Geometry: final body of the model. Coordinates: model frame, mm. A direction names the side the tool comes from. Give positions to 0.01 mm unless a question says otherwise; leave off trailing zeros. Write each loop counter-clockwise with the first axis right and the second up, starting at its lowest first coordinate (ties: lowest second). Pieces come first, ordered by that corner, then holes. Notation, with made-up numbers: (24, 5) - (39, 5) arc R8 ccw to (39, 17) - close; hole circle Ø11 at (-29.5, 36). An arc over 180 degrees is marked (long way). Return JSON: item names as keys, results as strings.
Autodesk Inventor part; units mm, degrees
ref_plane "Work Plane2" through (0, 0, -30) normal (0, 0, 1) x (1, 0, 0)
ref_plane "Work Plane3" through (45, 0, 0) normal (1, 0, 0) x (0, 1, 0)
ref_plane "XZ Plane" through (0, 0, 0) normal (0, 1, 0) x (-1, 0, 0)
sketch "Sketch1" plane through (0, 0, 0) normal (0, 1, 0) x (-1, 0, 0)
  line L0 (0, 0) -> (-90, 0)
  line L1 (-90, 0) -> (-90, -60)
  line L2 (-90, -60) -> (0, -60)
  line L3 (0, -60) -> (0, 0)
  line L4 (-30, 0) -> (-60, 0)
  line L5 (-60, 0) -> (-60, -60)
  line L6 (-60, -60) -> (-30, -60)
  line L7 (-30, -60) -> (-30, 0)
  line L8 (-20, -60) -> (-70, -60)
  line L9 (-70, -60) -> (-70, 0)
  line L10 (-70, 0) -> (-20, 0)
  line L11 (-20, 0) -> (-20, -60)
  line L12 (-20, -60) -> (-70, -60)
  line L13 (-70, -60) -> (-70, -40)
  line L14 (-70, -40) -> (-20, -40)
  line L15 (-20, -40) -> (-20, -60)
  circle A0 centre (-10, -50) radius 2.75
  circle A1 centre (-10, -10) radius 2.75
  circle A2 centre (-80, -50) radius 2.75
  circle A3 centre (-80, -10) radius 2.75
  point P0 (0, -30)
  point P1 (-60, -40)
  point P2 (-30, -40)
  point P3 (-70, 0)
  point P4 (-20, 0)
  dimension "d0" = 90
  dimension "d1" = 60
  dimension "d2" = 30
  dimension "d3" = 30
  dimension "d4" = 50
  dimension "d5" = 60
  dimension "d6" = 20
  dimension "d7" = 20
  dimension "d8" = 5.5
  dimension "d9" = 5.5
  dimension "d10" = 5.5
  dimension "d11" = 5.5
  dimension "d12" = 10
  dimension "d13" = 10
  dimension "d14" = 10
  dimension "d15" = 10
  dimension "d16" = 10
  dimension "d17" = 10
  dimension "d18" = 10
  dimension "d19" = 10
extrude "Extrusion1" add sketch "Sketch1" along normal blind 10 contours L3 L2 L11 L0 | L9 L2 L1 L0
extrude "Extrusion2" add sketch "Sketch1" along normal blind 20 contours L11 L14 L7 L0 | L7 L14 L5 L0 | L11 L2 L7 L14 | L5 L14 L9 L0 | L5 L2 L9 L14
extrude "Extrusion3" add sketch "Sketch1" along normal blind 50 contours L11 L2 L7 L14 | L7 L2 L5 L14 | L5 L2 L9 L14
extrude "Extrusion4" cut sketch "Sketch1" along normal blind 10 contours L7 L14 L5 L0 | L7 L2 L5 L14
ref_plane "Work Plane2" through (0, 0, -30) normal (0, 0, 1) x (1, 0, 0)
ref_plane "Work Plane3" through (45, 0, 0) normal (1, 0, 0) x (0, 1, 0)
sketch "Sketch7" plane through (0, 0, -30) normal (0, 0, 1) x (1, 0, 0)
  line L0 (20, 10) -> (20, 20)
  line L1 (20, 10) -> (0, 10)
  line L2 (20, 20) -> (0, 10)
  line L3 (0, 10) -> (20, 10)
  line L4 (20, 10) -> (20, 20)
  line L5 (70, 20) -> (60, 20)
  line L6 (70, 20) -> (90, 10)
  line L7 (90, 10) -> (70, 10)
  line L8 (90, 10) -> (70, 10)
  line L9 (70, 10) -> (70, 20)
  point P0 (0, 0)
extrude "Extrusion9" add sketch "Sketch7" along normal mid plane 4
sketch "Sketch8" plane through (45, 0, 0) normal (1, 0, 0) x (0, 1, 0)
  circle A0 centre (40, -50) radius 2.75
  line L0 (20, 0) -> (50, -51.9582)
  line L1 (20, 0) -> (20, -51.9582)
  line L2 (20, -51.9582) -> (50, -51.9582)
  point P0 (0, 0)
  point P1 (38.0692, -51.9582)
  point P2 (41.9308, -51.9582)
  dimension "d45" = 40
  dimension "d49" = 50
  dimension "d50" = 20
  dimension "d55" = 5.5
extrude "Extrusion10" add sketch "Sketch8" along normal mid plane 4 contours A0 L2 L1 L0
extrude "Extrusion11" cut sketch "Sketch8" along normal through all both and the other way through all contours A0 L2 | L2 A0
fillet "Fillet1" radius 10 2 edges at (45, 50, -40) (45, 50, -60)
properties part number "Homework 1d" material "Aluminum 6061"
Q1. Material intervals for probe 1 along Z at (x, y) = (10, 4.75); probe 2 along X at (y, z) = (7, -31.5); probe 3 along Z at (x, y) = (59, 40), sorted ascending. Write a range as [from, to].
Answer key:
{"probe 1": "z = [-60, -52.75], [-47.25, -12.75], [-7.25, 0]", "probe 2": "x = [0, 30], [60, 90]", "probe 3": "z = [-60, -52.75], [-47.25, -40]"}
Q2. Section query D-D, the plane z = -10. Return the cut outline in (x, y), plus the area to 3 significant figures.
Answer key:
{"outline": "(0, 0) - (7.25, 0) - (7.25, 10) - (0, 10) - close; (12.75, 0) - (30, 0) - (30, 10) - (60, 10) - (60, 0) - (77.25, 0) - (77.25, 10) - (70, 10) - (70, 20) - (47, 20) - (47, 25.77) - (43, 25.77) - (43, 20) - (20, 20) - (20, 10) - (12.75, 10) - close; (82.75, 0) - (90, 0) - (90, 10) - (82.75, 10) - close", "area": "1,010 mm^2"}
Q3. Mould query, pull axis Y, two halves, no side actions, for faces 6 (the flat face through (10, 15, -30)), 7 (the cylindrical face through (45.35, 37.973, -48.141)), 8 (the cylindrical face through (10.358, 4.93, -52.727)). Classes: pulls with the +Y half, pulls with the -Y half, needs draft (parallel to the pull), parting line crosses it, or undercut.
Answer key:
{"face 6": "pulls with the +Y half", "face 7": "undercut", "face 8": "needs draft"}
Q4. Pin query (flat end, axial travel): P1, Ø22.5, axis at y = 26, z = -46, coming from the +X side; P2, Ø6, axis at x = 54.5, y = 32.5, coming from the +Z side; P3, Ø11.5, axis at y = 26, z = -23.5, coming from the +X side. Return the tip coordinate at first contact, or that it passes through.
Answer key:
{"P1": "stops at x = 70", "P2": "stops at z = -40", "P3": "stops at x = 47"}
Q5. Set-up query: faces 1 (the flat face through (20, 25, -49)), 2 (the flat face through (30, 5, -30)), 3 (the flat face through (80, 10, -46)), 4 (the flat face through (32, 30, -40)), 5 (the flat face through (59, 30, -40)). Return all of +Z, -Z, +X, -X, +Y, -Y with unobstructed straight access to the full face (end or side cutting, diameter ignored); none if empty.
Answer key:
{"face 1": "-Z, -X, +Y", "face 2": "+Z, -Z, -Y", "face 3": "-Z, +X, +Y", "face 4": "+Z, -X, +Y", "face 5": "+Z, +X, +Y"}
Q6. Section query A-A, the plane y = 5. Return the cut outline in (x, z).
Answer key:
{"outline": "(0, -60) - (30, -60) - (30, 0) - (0, 0) - close; (60, -60) - (90, -60) - (90, 0) - (60, 0) - close; hole circle Ø5.5 at (10, -50); hole circle Ø5.5 at (10, -10); hole circle Ø5.5 at (80, -50); hole circle Ø5.5 at (80, -10)"}
Q7. Section query C-C, the plane x = 56. Return the cut outline in (y, z).
Answer key:
{"outline": "(10, -60) - (40, -60) arc R10 ccw to (40, -40) - (20, -40) - (20, 0) - (10, 0) - close; hole circle Ø5.5 at (40, -50)"}
Q8. Section query B-B, the plane x = 80. Return the cut outline in (y, z), plus the area to 3 significant figures.
Answer key:
{"outline": "(0, -60) - (10, -60) - (10, -52.75) - (0, -52.75) - close; (0, -47.25) - (10, -47.25) - (10, -32) - (15, -32) - (15, -28) - (10, -28) - (10, -12.75) - (0, -12.75) - close; (0, -7.25) - (10, -7.25) - (10, 0) - (0, 0) - close", "area": "510 mm^2"}
